Verification items for the finished model (mm, model axes). A direction names the side the tool comes from. Coordinates: 2 decimals unless noted, no trailing zeros. Order: outer loops, then holes, each group sorted by start corner. A loop starts at its lowest first (then second) coordinate and runs counter-clockwise, first axis right, second up. Notation, with made-up numbers: M 55,79.25 L 64,79.25 A32 ccw 64,110.25 Z; hole C -26.5,-28.75 d7. An arc over 180 degrees is marked long. Write item = value, one per line.
```python
from build123d import *

# Parameters (mm, degrees)
F1_DEPTH = 3
F3_DEPTH = 25
F5_DEPTH = 6
F6_SCALE = 0.5


with BuildPart() as f1:
    # F0 (on Top) → F1 (new body)
    with BuildSketch(Plane.XY):
        with BuildLine():
            ThreePointArc((69.1465082783, -7.3148026297), (69.4358131239, -3.6624855503), (69.532337402, 0))
            ThreePointArc((69.532337402, 0), (69.4358131239, 3.6624855503), (69.1465082783, 7.3148026297))
            ThreePointArc((69.1465082783, 7.3148026297), (49.1667872887, 49.1667872887), (7.3148026297, 69.1465082783))
            ThreePointArc((7.3148026297, 69.1465082783), (0, 69.532337402), (-7.3148026297, 69.1465082783))
            ThreePointArc((-7.3148026297, 69.1465082783), (-49.1667872887, 49.1667872887), (-69.1465082783, 7.3148026297))
            ThreePointArc((-69.1465082783, 7.3148026297), (-69.532337402, 0), (-69.1465082783, -7.3148026297))
            ThreePointArc((-69.1465082783, -7.3148026297), (-49.1667872887, -49.1667872887), (-7.3148026297, -69.1465082783))
            ThreePointArc((-7.3148026297, -69.1465082783), (0, -69.532337402), (7.3148026297, -69.1465082783))
            ThreePointArc((7.3148026297, -69.1465082783), (49.1667872887, -49.1667872887), (69.1465082783, -7.3148026297))
        make_face()
        with BuildLine():
            ThreePointArc((69.1465082783, 7.3148026297), (69.4358131239, 3.6624855503), (69.532337402, 0))
            ThreePointArc((69.532337402, 0), (69.4358131239, -3.6624855503), (69.1465082783, -7.3148026297))
            Line((69.1465082783, -7.3148026297), (87.8831749798, -7.3148026297))
            ThreePointArc((87.8831749798, -7.3148026297), (93.0555215223, -5.1723465425), (95.1979776095, 0))
            ThreePointArc((95.1979776095, 0), (93.0555215223, 5.1723465425), (87.8831749798, 7.3148026297))
            Line((87.8831749798, 7.3148026297), (69.1465082783, 7.3148026297))
        make_face()
        with BuildLine():
            ThreePointArc((-7.3148026297, 69.1465082783), (0, 69.532337402), (7.3148026297, 69.1465082783))
            Line((7.3148026297, 69.1465082783), (7.3148026297, 87.8831749798))
            ThreePointArc((7.3148026297, 87.8831749798), (5.1723465425, 93.0555215223), (0, 95.1979776095))
            ThreePointArc((0, 95.1979776095), (-5.1723465425, 93.0555215223), (-7.3148026297, 87.8831749798))
            Line((-7.3148026297, 87.8831749798), (-7.3148026297, 69.1465082783))
        make_face()
        with BuildLine():
            Line((7.3148026297, -87.8831749798), (7.3148026297, -69.1465082783))
            ThreePointArc((7.3148026297, -69.1465082783), (0, -69.532337402), (-7.3148026297, -69.1465082783))
            Line((-7.3148026297, -69.1465082783), (-7.3148026297, -87.8831749798))
            ThreePointArc((-7.3148026297, -87.8831749798), (-5.1723465425, -93.0555215223), (0, -95.1979776095))
            ThreePointArc((0, -95.1979776095), (5.1723465425, -93.0555215223), (7.3148026297, -87.8831749798))
        make_face()
        with BuildLine():
            ThreePointArc((-69.1465082783, -7.3148026297), (-69.532337402, 0), (-69.1465082783, 7.3148026297))
            Line((-69.1465082783, 7.3148026297), (-87.8831749798, 7.3148026297))
            ThreePointArc((-87.8831749798, 7.3148026297), (-93.0555215223, 5.1723465425), (-95.1979776095, 0))
            ThreePointArc((-95.1979776095, 0), (-93.0555215223, -5.1723465425), (-87.8831749798, -7.3148026297))
            Line((-87.8831749798, -7.3148026297), (-69.1465082783, -7.3148026297))
        make_face()
    extrude(amount=F1_DEPTH)

    # F2 (on face) → F3 (cut)
    with BuildSketch(Plane.XY.offset(3)):
        with BuildLine():
            Line((16.5183525532, 18.4991825372), (28.2446611673, 30.4242391139))
            ThreePointArc((28.2446611673, 30.4242391139), (-6.7759205764, 40.1934215699), (-35.9519049525, 18.4991825372))
            Line((-35.9519049525, 18.4991825372), (-22.1387110651, 7.7666295692))
            ThreePointArc((-22.1387110651, 7.7666295692), (-5.7075669458, 23.5688666851), (16.5183525532, 18.4991825372))
        make_face()
        with BuildLine():
            Line((0.6598568289, -8.2568302751), (22.8720060756, -8.2568302751))
            ThreePointArc((22.8720060756, -8.2568302751), (20.6804420753, -14.1282137838), (16.8557025786, -19.0928351043))
            Line((16.8557025786, -19.0928351043), (29.8348077707, -28.9163588455))
            ThreePointArc((29.8348077707, -28.9163588455), (30.1844763243, -28.5097115536), (30.5290018042, -28.0986977933))
            ThreePointArc((30.5290018042, -28.0986977933), (39.0530735531, -11.2241482879), (39.4424125552, 7.6771383174))
            Line((39.4424125552, 7.6771383174), (0.6598568289, 7.6771383174))
            Line((0.6598568289, 7.6771383174), (0.6598568289, -8.2568302751))
        make_face()
        with BuildLine():
            ThreePointArc((-21.936269477, -7.7693820931), (-23.5046233838, -1.3017309627), (-22.9253014498, 5.3280979354))
            Line((-22.9253014498, 5.3280979354), (-37.0819843029, 16.0259236856))
            ThreePointArc((-37.0819843029, 16.0259236856), (-40.272638067, -1.3002890528), (-35.9932072461, -18.3901805431))
            Line((-35.9932072461, -18.3901805431), (-21.936269477, -7.7693820931))
        make_face()
        with BuildLine():
            Line((-21.0756994649, -10.0013930179), (-34.6712230282, -20.7951781903))
            ThreePointArc((-34.6712230282, -20.7951781903), (-5.653058159, -40.5104727569), (28.0658900738, -30.8265034109))
            Line((28.0658900738, -30.8265034109), (14.7211225703, -20.8851005882))
            ThreePointArc((14.7211225703, -20.8851005882), (-5.6704095402, -23.6431925936), (-21.0756994649, -10.0013930179))
        make_face()
    extrude(amount=-F3_DEPTH, mode=Mode.SUBTRACT)

    # F4 (on face) → F5 (join)
    with BuildSketch(Plane.XY.offset(3)):
        with BuildLine():
            Line((16.5639953805, 15.693101771), (31.1080969783, 30.4837098063))
            ThreePointArc((31.1080969783, 30.4837098063), (-6.9286387342, 42.198718121), (-38.464639275, 17.9187808608))
            Line((-38.464639275, 17.9187808608), (-38.4463550975, 17.9045744503))
            Line((-38.4463550975, 17.9045744503), (-21.0883413572, 4.4177731062))
            Line((-21.0883413572, 4.4177731062), (-20.9411330852, 4.303395462))
            ThreePointArc((-20.9411330852, 4.303395462), (-5.6797522011, 21.4943554028), (16.5639953805, 15.693101771))
        make_face()
        with BuildLine():
            ThreePointArc((-35.9519049525, 18.4991825372), (-6.7759205764, 40.1934215699), (28.2446611673, 30.4242391139))
            Line((28.2446611673, 30.4242391139), (16.5183525532, 18.4991825372))
            ThreePointArc((16.5183525532, 18.4991825372), (-5.7075669458, 23.5688666851), (-22.1387110651, 7.7666295692))
            Line((-22.1387110651, 7.7666295692), (-35.9519049525, 18.4991825372))
        make_face(mode=Mode.SUBTRACT)
        with BuildLine():
            Line((-19.5500680933, -8.473156722), (-36.6423058309, -21.3872931472))
            ThreePointArc((-36.6423058309, -21.3872931472), (-4.9960373644, -42.6296318895), (31.1903517483, -30.6601496082))
            Line((31.1903517483, -30.6601496082), (31.0539440179, -30.5585304384))
            ThreePointArc((31.0539440179, -30.5585304384), (30.573900942, -31.0902940329), (30.0853848234, -31.6142843735))
            Line((30.0853848234, -31.6142843735), (13.66533039, -19.1864018522))
            ThreePointArc((13.66533039, -19.1864018522), (-5.4535220983, -21.615371302), (-19.5500680933, -8.473156722))
        make_face()
        with BuildLine():
            ThreePointArc((-21.0756994649, -10.0013930179), (-5.6704095402, -23.6431925936), (14.7211225703, -20.8851005882))
            Line((14.7211225703, -20.8851005882), (28.0658900738, -30.8265034109))
            ThreePointArc((28.0658900738, -30.8265034109), (-5.653058159, -40.5104727569), (-34.6712230282, -20.7951781903))
            Line((-34.6712230282, -20.7951781903), (-21.0756994649, -10.0013930179))
        make_face(mode=Mode.SUBTRACT)
        with BuildLine():
            Line((-21.0883413572, 4.4177731062), (-38.4463550975, 17.9045744503))
            ThreePointArc((-38.4463550975, 17.9045744503), (-42.2485928064, -1.9617758618), (-36.6614406796, -21.4017505898))
            Line((-36.6614406796, -21.4017505898), (-36.6423058309, -21.3872931472))
            ThreePointArc((-36.6423058309, -21.3872931472), (-36.9523718103, -20.8420801294), (-37.2545148762, -20.2924368686))
            Line((-37.2545148762, -20.2924368686), (-20.1947009372, -6.7482753745))
            ThreePointArc((-20.1947009372, -6.7482753745), (-21.5038361154, -1.2342638661), (-21.0883413572, 4.4177731062))
        make_face()
        with BuildLine():
            Line((-21.936269477, -7.7693820931), (-35.9932072461, -18.3901805431))
            ThreePointArc((-35.9932072461, -18.3901805431), (-40.272638067, -1.3002890528), (-37.0819843029, 16.0259236856))
            Line((-37.0819843029, 16.0259236856), (-22.9253014498, 5.3280979354))
            ThreePointArc((-22.9253014498, 5.3280979354), (-23.5046233838, -1.3017309627), (-21.936269477, -7.7693820931))
        make_face(mode=Mode.SUBTRACT)
        with BuildLine():
            ThreePointArc((-20.0629168504, -7.0638754616), (-20.1295357126, -6.9063789134), (-20.1947009372, -6.7482753745))
            Line((-20.1947009372, -6.7482753745), (-37.2545148762, -20.2924368686))
            ThreePointArc((-37.2545148762, -20.2924368686), (-36.9523718103, -20.8420801294), (-36.6423058309, -21.3872931472))
            Line((-36.6423058309, -21.3872931472), (-19.5500680933, -8.473156722))
            ThreePointArc((-19.5500680933, -8.473156722), (-19.8181327724, -7.7727520906), (-20.0629168504, -7.0638754616))
        make_face()
        with BuildLine():
            ThreePointArc((14.778628294, -18.4339677859), (14.2275475814, -18.8184235598), (13.66533039, -19.1864018522))
            Line((13.66533039, -19.1864018522), (30.0853848234, -31.6142843735))
            ThreePointArc((30.0853848234, -31.6142843735), (30.573900942, -31.0902940329), (31.0539440179, -30.5585304384))
            Line((31.0539440179, -30.5585304384), (14.778628294, -18.4339677859))
        make_face()
        with BuildLine():
            Line((13.660088258, -19.1824342282), (13.66533039, -19.1864018522))
            ThreePointArc((13.66533039, -19.1864018522), (14.2275475814, -18.8184235598), (14.778628294, -18.4339677859))
            Line((14.778628294, -18.4339677859), (31.0539440179, -30.5585304384))
            ThreePointArc((31.0539440179, -30.5585304384), (41.0029367993, -11.6707107453), (41.0420586495, 9.6771383174))
            Line((41.0420586495, 9.6771383174), (-1.3401431711, 9.6771383174))
            Line((-1.3401431711, 9.6771383174), (-1.3401431711, -10.2568302751))
            Line((-1.3401431711, -10.2568302751), (20.238117635, -10.2568302751))
            ThreePointArc((20.238117635, -10.2568302751), (17.6137295695, -15.2094515931), (13.660088258, -19.1824342282))
        make_face()
        with BuildLine():
            Line((0.6598568289, -8.2568302751), (0.6598568289, 7.6771383174))
            Line((0.6598568289, 7.6771383174), (39.4424125552, 7.6771383174))
            ThreePointArc((39.4424125552, 7.6771383174), (38.9201464557, -11.7437255239), (29.8348077707, -28.9163588455))
            Line((29.8348077707, -28.9163588455), (16.8557025786, -19.0928351043))
            ThreePointArc((16.8557025786, -19.0928351043), (20.6804420753, -14.1282137838), (22.8720060756, -8.2568302751))
            Line((22.8720060756, -8.2568302751), (0.6598568289, -8.2568302751))
        make_face(mode=Mode.SUBTRACT)
    extrude(amount=F5_DEPTH)


with BuildPart() as f1_1:
    # F6: moved
    add(f1.part.scale(F6_SCALE))


solid = f1_1.part
```
Item 1: Release check for a two-part mould opening along Y. For faces 6 (the cylindrical face through (-3.18, 21.15, 2.98)), 7 (the cylindrical face through (-2.69, 11.83, 2.22)), 8 (the flat face through (0.33, 0, 2)), 9 (the flat face through (0, 0, 4.5)) record: pulls with the +Y half, pulls with the -Y half, needs draft (parallel to the pull), parting line crosses it, or undercut.
Report:
face_6 = pulls with the +Y half
face_7 = undercut
face_8 = undercut
face_9 = needs draft
Item 2: Gauge pin test, flat ends, axial feed: pin 1 (1.5 mm diameter, centred on x = 14, z = 2, fed in from +Y); pin 2 (2 mm diameter, centred on x = -26.5, z = 1.5, fed in from -Y); pin 3 (1.2 mm diameter, centred on y = -39.5, z = 1, fed in from -X). Record the tip position at first contact, or that the pin passes through.
Report:
pin_1 = 32.06
pin_2 = -23.63
pin_3 = -3.66
Item 3: Sectioned sample at A-A, the plane x = 2. Enter the section's corners in (y, z).
Report:
outline = M -47,0 L -20.46,0 L -20.46,4.5 L -21.46,4.5 L -21.46,1.5 L -47,1.5 Z; M -12.29,0 L -4.13,0 L -4.13,4.5 L -5.13,4.5 L -5.13,1.5 L -11.29,1.5 L -11.29,4.5 L -12.29,4.5 Z; M 3.84,0 L 12.11,0 L 12.11,4.5 L 11.1,4.5 L 11.1,1.5 L 4.84,1.5 L 4.84,4.5 L 3.84,4.5 Z; M 20.38,0 L 47,0 L 47,1.5 L 21.38,1.5 L 21.38,4.5 L 20.38,4.5 Z
Item 4: Tool access check on faces 1 (the cylindrical face through (-3.647, 20.047, 2.218)), 2 (the cylindrical face through (20.465, -5.982, 2.979)), 3 (the flat face through (-0.67, 0, 3)), 4 (the flat face through (-1, 1, 0)), 5 (the cylindrical face through (-24.348, 24.816, 0.74)). Record the directions out of +Z, -Z, +X, -X, +Y, -Y that give a thin tool (end or side, any length) a straight path to the whole face; none if there is none.
Report:
face_1 = +Z, -Z
face_2 = +Z, +X
face_3 = +Z
face_4 = -Z, +X, -X, +Y, -Y
face_5 = +Z, -Z, -X, +Y
Item 5: Sectioned sample at B-B, the plane y = -39.5. Enter the section's corners in (x, z), then the cut area to 3 significant figures.
Report:
outline = M -3.66,0 L 3.66,0 L 3.66,1.5 L -3.66,1.5 Z
area = 11.0 mm^2
Item 6: Sectioned sample at D-D, the plane x = -15. Enter the section's corners in (y, z), then the cut area to 3 significant figures.
Report:
outline = M -31.36,0 L -13.59,0 L -13.59,4.5 L -15.05,4.5 L -15.05,1.5 L -31.36,1.5 Z; M -8.54,0 L -6.93,0 L -6.93,4.5 L -8.54,4.5 Z; M 5.34,0 L 6.94,0 L 6.94,4.5 L 5.34,4.5 Z; M 13.57,0 L 31.36,0 L 31.36,1.5 L 15.03,1.5 L 15.03,4.5 L 13.57,4.5 Z
area = 76.6 mm^2
Item 7: Scan lines: L1, parallel to Y at x = -12, z = 2; L2, parallel to Y at x = 8, z = 2.5; L3, parallel to X at y = -13, z = 3.1. Record each from-to range of solid material in increasing order. Write a range as from..to.
Report:
L1 = -17.59..-16.35, -6.16..-4.66, 3.07..4.61, 16.32..17.55
L2 = -20.15..-19.08, -10.92..-8.56, -5.13..-4.13, 3.84..4.84, 8.13..9.47, 18.99..20.06
L3 = -16.78..-15.51, 10.79..12.99, 16.08..17.3
